Model file for the job. Use its own axes, mm. Face numbers are marked on the shaded views. Give positions to 0.01 mm unless a question says otherwise; leave off trailing zeros. Order: outer loops, then holes, each group sorted by start corner. A loop starts at its lowest first (then second) coordinate and runs counter-clockwise, first axis right, second up. Notation, with made-up numbers: (82, -34.75) - (131, -34.75) arc R20 cw to (131, -18.75) - close; hole circle Ø7 at (50.25, 75). An arc over 180 degrees is marked (long way). Use CSV: the item, a comma, the result in double quotes. Start each with the question number.
(1) Band-saw the part on B-B, the plane y = 9. Give the cut face in (x, z), then the cut area to 3 significant figures.
(2) Drop a flat-ended pin along its axis: pin 1 Ø2.5 at (x, z) = (4.35, 5.78) entering from -Y. Give the stop position or say it passes through.
(3) Band-saw the part on C-C, the plane z = 5.5. Give the cut face in (x, y).
(4) Probe L1, parallel to X at y = 1, z = 7; L2, parallel to X at y = 9.25, z = 6.25; L3, parallel to X at y = 10.25, z = 7.75. List the from-to ranges inside material, lowest first.
(5) Band-saw the part on A-A, the plane x = 13. Give the cut face in (y, z), then the cut area to 3 significant figures.
(6) Pull direction X, two halves, no side cores. Call the marked faces 1, 2 and 3: +X half, -X half, draft (parallel to the pull), parting line (faces both ways), or undercut.
(7) Band-saw the part on D-D, the plane x = 5.5. Give the cut face in (y, z), then the cut area to 3 significant figures.
from build123d import *

# Parameters (mm, degrees)
SKETCH_1_W        = 18.8
SKETCH_1_H        = 8
EXTRUDE_1_DEPTH   = 10.5
FILLET_1_R        = 1
HOLE_WIZARD_M31_D = 3.4


with BuildPart() as part:
    # Эскиз1 → Бобышка-Вытянуть1 (new body)
    with BuildSketch(Plane(origin=(0, 0, 0), x_dir=(1, 0, 0), z_dir=(0, 1, 0))):
        with Locations((9.4, -4)):
            Rectangle(SKETCH_1_W, SKETCH_1_H)
    extrude(amount=EXTRUDE_1_DEPTH)

    # Скругление1
    fillet_1_edges = [part.edges().sort_by_distance(p)[0] for p in [
        (18.8, 5.25, 8),
        (0, 5.25, 8),
    ]]
    fillet(fillet_1_edges, radius=FILLET_1_R)

    # Отверстие с зазором M31 (through all)
    with Locations(Plane(origin=(0, 10.5, 0), x_dir=(1, 0, 0), z_dir=(0, 1, 0))):
        with Locations((4.350247301, -5.779226371), (14.350247301, -5.779226371)):
            Hole(HOLE_WIZARD_M31_D / 2)


solid = part.part
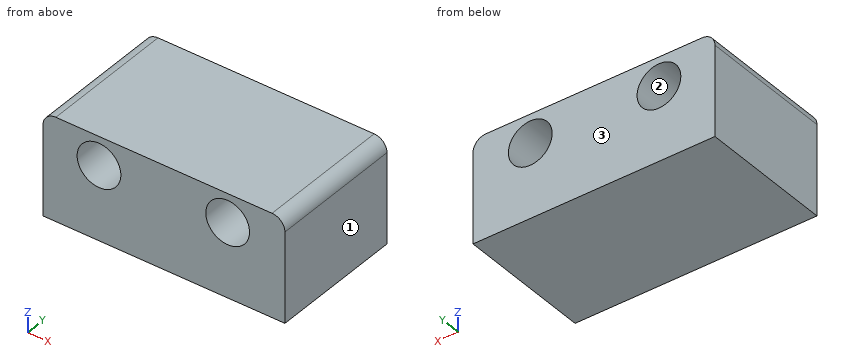
Answer block:
1,outline,"(0, 0) - (18.8, 0) - (18.8, 7) arc R1 ccw to (17.8, 8) - (1, 8) arc R1 ccw to (0, 7) - close; hole circle Ø3.4 at (4.35, 5.78); hole circle Ø3.4 at (14.35, 5.78)"
1,area,"132 mm2"
2,pin 1,"passes through"
3,outline,"(0, 0) - (2.67, 0) - (2.67, 10.5) - (0, 10.5) - close; (6.03, 0) - (12.67, 0) - (12.67, 10.5) - (6.03, 10.5) - close; (16.03, 0) - (18.8, 0) - (18.8, 10.5) - (16.03, 10.5) - close"
4,L1,"x = 0 to 3.17, 5.53 to 13.17, 15.53 to 18.8"
4,L2,"x = 0 to 2.72, 5.98 to 12.72, 15.98 to 18.8"
4,L3,"x = 0.34 to 18.46"
5,outline,"(0, 0) - (10.5, 0) - (10.5, 4.75) - (0, 4.75) - close; (0, 6.81) - (10.5, 6.81) - (10.5, 8) - (0, 8) - close"
5,area,"62.3 mm2"
6,face 1,"+X half"
6,face 2,"undercut"
6,face 3,"draft"
7,outline,"(0, 0) - (10.5, 0) - (10.5, 4.53) - (0, 4.53) - close; (0, 7.03) - (10.5, 7.03) - (10.5, 8) - (0, 8) - close"
7,area,"57.7 mm2"
